Autodesk Inventor part; units mm, degrees
ref_plane "YZ Plane" through (0, 0, 0) normal (1, 0, 0) x (0, 1, 0)
ref_plane "XZ Plane" through (0, 0, 0) normal (0, 1, 0) x (-1, 0, 0)
ref_plane "XY Plane" through (0, 0, 0) normal (0, 0, 1) x (1, 0, 0)
sketch "Sketch1" plane through (0, 0, 0) normal (0, 0, 1) x (1, 0, 0)
  line L0 (-115.1754, 107.4561) -> (0.7036, 107.4561)
  line L1 (0.7036, 107.4561) -> (0.7036, 5.8561)
  line L2 (0.7036, 5.8561) -> (-115.1754, 5.8561)
  line L3 (-115.1754, 5.8561) -> (-115.1754, 107.4561)
  line L4 (-115.1754, 107.4561) -> (-100.8964, 5.8561)
  arc A0 (-105.5234, 107.4561) -> (0.7036, 15.5081) centre (6.6, 129.6559) ccw
  line L5 (-101.9706, 13.4992) -> (-91.8279, 5.8561)
  dimension "d0" = 101.6
  dimension "d2" = 8
  dimension "d6" = 9.652
  dimension "d7" = 9.652
  dimension "d8" = 114.3
  dimension "d9" = 123.7998
  dimension "d13" = 101.6
  dimension "d14" = 12.7
  dimension "d15" = 37
extrude "Extrusion1" add sketch "Sketch1" along normal blind 6.35 contours L0 A0 L1 L2 L5 L4
properties part number "FE-00013-03"
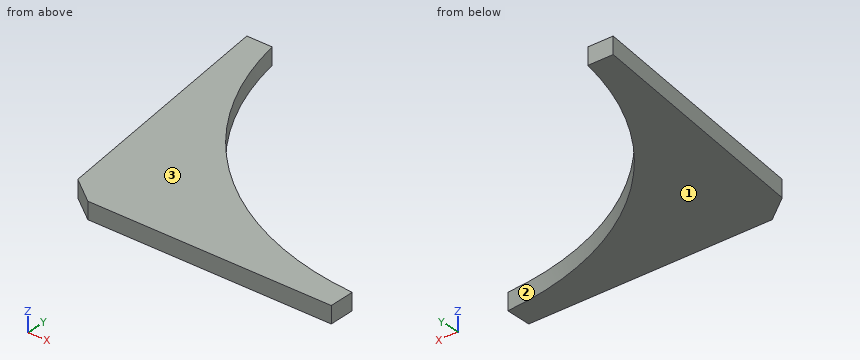
Build history of the part. All positions in model axes, mm. Face numbers are marked on the shaded views. Round coordinates to 2 decimals unless told otherwise and drop trailing zeros. Loops run counter-clockwise (first coordinate to the right, second up) from the corner with the lowest first, then second, coordinate; pieces in that order, holes last.
Item 1: Saw through at B-B (x = -60). List the corners of the cut face in (y, z), then the cut area to 3 significant figures.
Item 2: Two-plate mould, pull along Z, no slides. Class the marked faces 1, 2 and 3: released by +Z, released by -Z, zero draft, split by the parting line, or undercut.
Item 3: Drill centre lines: line 1 along X through (y, z) = (89, 3.5); line 2 along X through (y, z) = (59, 2); line 3 along Y through (x, z) = (-32.5, 2). Where is each one in solid material? Low to high.
Item 4: Saw through at C-C (y = 35). List the corners of the cut face in (x, z), then the cut area to 3 significant figures.
Item 5: Saw through at A-A (z = 1). List the corners of the cut face in (x, y), then the cut area to 3 significant figures.
Item 6: Pin check, flat tips, straight feed: P1, Ø2, axis at y = 48, z = 5, coming from the -X side; P2, Ø1.5, axis at y = 49.5, z = 3, coming from the +X side. Stop position of each tip, or through.
Worked answers:
1. outline: (5.86, 0) - (36.76, 0) - (36.76, 6.35) - (5.86, 6.35) - close
1. area: 196 mm2
2. face 1: released by -Z
2. face 2: zero draft
2. face 3: released by +Z
3. line 1: x = -112.58 to -100.23
3. line 2: x = -108.37 to -83.25
3. line 3: y = 5.86 to 22.25
4. outline: (-104.99, 0) - (-57.47, 0) - (-57.47, 6.35) - (-104.99, 6.35) - close
4. area: 302 mm2
5. outline: (-115.18, 107.46) - (-101.97, 13.5) - (-91.83, 5.86) - (0.7, 5.86) - (0.7, 15.51) arc R114.3 cw to (-105.52, 107.46) - close
5. area: 3,820 mm2
6. P1: stops at x = -106.96
6. P2: stops at x = -74.14
